Design review of the part shown in the three views and the two pictorial views. Dimensions are in mm from the part's minimum x, y and z. A direction names the side the tool comes from. Round coordinates to 2 decimals unless told otherwise and drop trailing zeros. Order: outer loops, then holes, each group sorted by start corner. A loop starts at its lowest first (then second) coordinate and runs counter-clockwise, first axis right, second up. Notation, with made-up numbers: (71, 88) - (102, 88) arc R19 ccw to (102, 111) - close; hole circle Ø11 at (26, 72.5). An arc over 180 degrees is marked (long way). One line per item, written item: value.
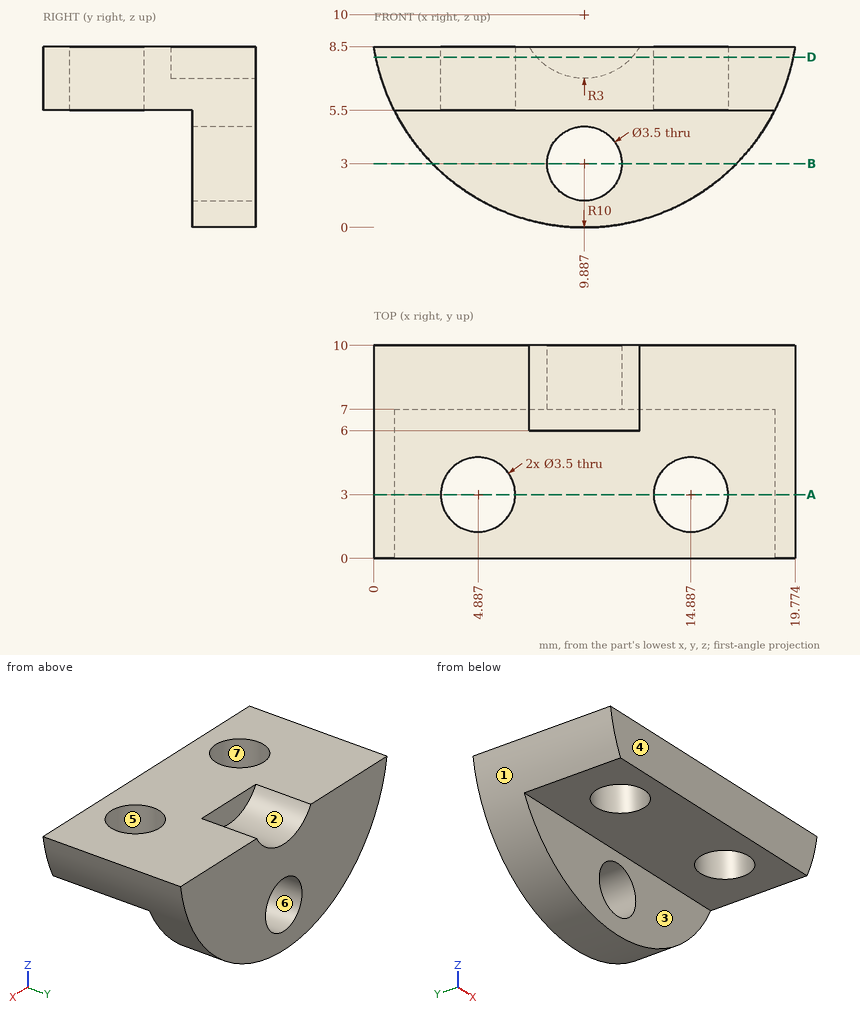
Item 1: Wall thickness on line 1 (Y direction, x = 5, z = 6.5); line 2 (X direction, y = 3.75, z = 8.25) (1 decimal); line 3 (Y direction, x = 15.75, z = 2.75): over which ranges is each line inside the solid? List them lowest first.
Returned:
line 1: 0 to 1.25, 4.75 to 10
line 2: 0 to 3.3, 6.5 to 13.3, 16.5 to 19.7
line 3: 7 to 10
Item 2: Take a section at B-B (z = 3). Write out the cut boundary in (x, y) (1 decimal).
Returned:
outline: (2.7, 7) - (8.1, 7) - (8.1, 10) - (2.7, 10) - close; (11.6, 7) - (17, 7) - (17, 10) - (11.6, 10) - close
Item 3: Machinability: for the marked faces 1, 2 and 3, which of the approach directions +Z, -Z, +X, -X, +Y, -Y give a long, thin tool a straight path to every point of the face, cutting with its end or side? Answer none if there is none.
Returned:
face 1: -Z, +Y, -Y
face 2: +Z, +Y
face 3: -Z, +X, -X, -Y
Item 4: Take a section at D-D (z = 8). Count the separate pieces of the cut face and the enclosed holes in it, plus the area to 3 significant figures.
Returned:
separate pieces: 1
enclosed holes: 2
area: 159 mm^2
Item 5: For P1, Ø3, axis at x = 14.89, y = 3, coming from the -Z side; P2, Ø1, axis at y = 7, z = 3.5, coming from the -X side; P3, Ø3, axis at x = 8, z = 3, coming from the -Y side; P4, Ø2, axis at x = 13.5, y = 3, coming from the -Z side, all flat-tipped, find the tip position at first contact; note any pin that passes through.
Returned:
P1: through
P2: x = 1.89
P3: y = 7
P4: z = 5.5
Item 6: Take a section at A-A (y = 3). Write out the cut boundary in (x, z).
Returned:
outline: (0, 8.5) arc R10 ccw to (0.96, 5.5) - (3.14, 5.5) - (3.14, 8.5) - close; (6.64, 5.5) - (13.14, 5.5) - (13.14, 8.5) - (6.64, 8.5) - close; (16.64, 5.5) - (18.82, 5.5) arc R10 ccw to (19.77, 8.5) - (16.64, 8.5) - close
Item 7: The part is to be moulded in two halves that separate along Y. For the marked faces 4, 5, 6 and 7, say which applies: +Y half, -Y half, draft (parallel to the pull), parting line (faces both ways), or undercut.
Returned:
face 4: -Y half
face 5: undercut
face 6: draft
face 7: undercut
